```python
from build123d import *

# Parameters (mm, degrees)
RESSALTO_EXTRUS_O1_DEPTH = 50


with BuildPart() as part:
    # Esboço1 → Ressalto-extrusão1 (new, symmetric)
    with BuildSketch(Plane(origin=(0, 0, 0), x_dir=(0, 0, -1), z_dir=(1, 0, 0))):
        with BuildLine():
            Line((12.814923667, -40.354099314), (20.74666802, -39.311299471))
            ThreePointArc((20.74666802, -39.311299471), (38.065679381, -22.952266843), (44.45, 0))
            Line((44.45, 0), (44.45, 28.878170812))
            Line((44.45, 28.878170812), (42.34, 28.878170812))
            Line((42.34, 28.878170812), (42.34, 0))
            ThreePointArc((42.34, 0), (34.170597508, -25.000917303), (12.814923667, -40.354099314))
        make_face()
    extrude(amount=RESSALTO_EXTRUS_O1_DEPTH, both=True)


solid = part.part
```
Model file for the job. Use its own axes, mm. A direction names the side the tool comes from. Give positions to 0.01 mm unless a question says otherwise; leave off trailing zeros. Order: outer loops, then holes, each group sorted by start corner. A loop starts at its lowest first (then second) coordinate and runs counter-clockwise, first axis right, second up.
1) Saw through at A-A, the plane y = 15. Write the cut outline in (x, z), then the cut area to 3 significant figures.
2) 3-axis set-ups, long thin cutter, end or side, ignore diameter. For faces 1 (the flat face through (1, 15, -42.34)), 2 (the flat face through (1, 28.878, -43)): which of +Z, -Z, +X, -X, +Y, -Y reach the whole face in a straight line?
3) Pin check, flat tips, straight feed: pin 1 (10 mm diameter, centred on x = -23, y = -11, fed in from +Z); pin 2 (3 mm diameter, centred on x = -31, y = 2, fed in from +Z); pin 3 (2 mm diameter, centred on x = 28, z = -33.5, fed in from -Y). Stop position of each tip, or through.
4) Saw through at B-B, the plane x = -28. Write the cut outline in (y, z), then the cut area to 3 significant figures.
5) Saw through at C-C, the plane z = -35.5. Write the cut outline in (x, y), then the cut area to 3 significant figures.
6) Wall check: probe 1 along Z at (x, y) = (7.5, 16.5); probe 2 along Y at (x, z) = (35, -33.5); probe 3 along Z at (x, y) = (-3.5, -7). Give the ranges that are in metal, low to high.
Computed:
1. outline: (-50, -44.45) - (50, -44.45) - (50, -42.34) - (-50, -42.34) - close
1. area: 211 mm2
2. face 1: +Z, +X, -X, +Y
2. face 2: +Z, -Z, +X, -X, +Y
3. pin 1: stops at z = -39.2
3. pin 2: stops at z = -42.34
3. pin 3: stops at y = -30.32
4. outline: (-40.35, -12.81) - (-39.31, -20.75) arc R44.45 ccw to (0, -44.45) - (28.88, -44.45) - (28.88, -42.34) - (0, -42.34) arc R42.34 cw to start
4. area: 167 mm2
5. outline: (-50, -26.75) - (50, -26.75) - (50, -23.07) - (-50, -23.07) - close
5. area: 368 mm2
6. probe 1: z = -44.45 to -42.34
6. probe 2: y = -29.22 to -25.89
6. probe 3: z = -43.9 to -41.76
